Build history of the part. All positions in model axes, mm. A direction names the side the tool comes from. Round coordinates to 2 decimals unless told otherwise and drop trailing zeros. Write each loop counter-clockwise with the first axis right and the second up, starting at its lowest first coordinate (ties: lowest second). Pieces come first, ordered by that corner, then holes. Notation, with made-up numbers: (-7, 85) - (42, 85) arc R8 cw to (42, 93) - close; hole circle Ø3 at (61, 52.25). An arc over 180 degrees is marked (long way). Answer as a JSON object with one key per item and string values. Group by question number.
Item 1: Slice it at A-A, the plane y = 11. List the corners of the cut face in (x, z), then the cut area to 3 significant figures.
Item 2: Flat gauge pins, fed straight in: pin 1 (3.5 mm diameter, centred on x = 11, y = 0, fed in from -Z); pin 2 (8 mm diameter, centred on x = 2, y = -0.5, fed in from +Z); pin 3 (3.5 mm diameter, centred on x = -11, y = 0, fed in from +Z); pin 4 (1.5 mm diameter, centred on x = -5.5, z = 0.5, fed in from +Y). Where does each tip first touch, or does it go through?
Item 3: Probe line 1 (Y direction, x = 0, z = 1.1); line 2 (Y direction, x = -1.5, z = 2.15); line 3 (Y direction, x = -8.75, z = 0.35). List the from-to ranges inside material, lowest first. Write a range as from..to.
Item 4: Two-plate mould, pull along Y, no slides. Class faces 1 (the flat face through (6, 0, 3)), 2 (the cylindrical face through (-14.985, 0.66, 1.479)), 3 (the cylindrical face through (-0.54, 13.44, 1.24)): +Y half, -Y half, draft (parallel to the pull), parting line (faces both ways), or undercut.
Item 5: Which spindle directions (+Z, -Z, +X, -X, +Y, -Y) get a long thin tool onto all of the face, cutting with end or side? Do faces 4 (the cylindrical face through (-1.08, -4.88, 2.25)), 5 (the cylindrical face through (-0.54, -8.56, 1.24)), 6 (the cylindrical face through (-0.54, -2.44, 1.01)). Say none if no direction does.
Item 6: Slice it at C-C, the plane y = 0. Give the number of separate pieces and of enclosed holes in the cut face, then the cut area to 3 significant figures.
from build123d import *

# Parameters (mm, degrees)
SKETCH_R        = 15
SKETCH_R_2      = 1.5
PAD_DEPTH       = 3
SKETCH002_R     = 2.5
POCKET_DEPTH    = 9
SKETCH001_R     = 5
POCKET001_DEPTH = 1
SKETCH003_R     = 2.5
POCKET002_DEPTH = 2
CHAMFER_SIZE    = 0.5
CHAMFER001_SIZE = 0.4


with BuildPart() as part:
    # Sketch → Pad (new body)
    with BuildSketch(Plane.XY):
        Circle(SKETCH_R)
        with Locations((0, 11)):
            Circle(SKETCH_R_2, mode=Mode.SUBTRACT)
        with Locations((-11, 0)):
            Circle(SKETCH_R_2, mode=Mode.SUBTRACT)
        with Locations((0, -11)):
            Circle(SKETCH_R_2, mode=Mode.SUBTRACT)
        with Locations((11, 0)):
            Circle(SKETCH_R_2, mode=Mode.SUBTRACT)
    extrude(amount=PAD_DEPTH)

    # Sketch002 (on Face7 of Pad) → Pocket (cut)
    with BuildSketch(Plane.XY.offset(3)):
        Circle(SKETCH002_R)
    extrude(amount=-POCKET_DEPTH, mode=Mode.SUBTRACT)

    # Sketch001 (on Face7 of Pad) → Pocket001 (cut)
    with BuildSketch(Plane.XY.offset(3)):
        Circle(SKETCH001_R)
    extrude(amount=-POCKET001_DEPTH, mode=Mode.SUBTRACT)

    # Sketch003 (on Face2 of Pocket001) → Pocket002 (cut)
    with BuildSketch(Plane(origin=(0, 0, 0), x_dir=(1, 0, 0), z_dir=(0, 0, -1))):
        with Locations((0, 11)):
            Circle(SKETCH003_R)
        with Locations((11, 0)):
            Circle(SKETCH003_R)
        with Locations((0, -11)):
            Circle(SKETCH003_R)
        with Locations((-11, 0)):
            Circle(SKETCH003_R)
    extrude(amount=-POCKET002_DEPTH, mode=Mode.SUBTRACT)

    # Chamfer
    chamfer_edges = [part.edges().sort_by_distance(p)[0] for p in [
        (-1.5, 11, 3),
        (9.5, 0, 3),
        (-1.5, -11, 3),
        (-12.5, 0, 3),
        (-5, 0, 3),
        (-2.5, 0, 2),
        (-2.5, -11, 0),
        (8.5, 0, 0),
        (-2.5, 11, 0),
        (-13.5, 0, 0),
        (-2.5, 0, 0),
    ]]
    chamfer(chamfer_edges, length=CHAMFER_SIZE)

    # Chamfer001
    chamfer001_edges = [part.edges().sort_by_distance(p)[0] for p in [
        (-1.5, -11, 2),
        (9.5, 0, 2),
        (-1.5, 11, 2),
        (-12.5, 0, 2),
    ]]
    chamfer(chamfer001_edges, length=CHAMFER001_SIZE)


solid = part.part
Geometry says:
{
 "1": {"outline": "(-10.2, 0) - (-3, 0) - (-2.5, 0.5) - (-2.5, 2) - (-1.9, 2) - (-1.5, 2.4) - (-1.5, 2.5) - (-2, 3) - (-10.2, 3) - close; (1.5, 2.4) - (1.9, 2) - (2.5, 2) - (2.5, 0.5) - (3, 0) - (10.2, 0) - (10.2, 3) - (2, 3) - (1.5, 2.5) - close", "area": "47.5 mm^2"},
 "2": {"pin 1": "stops at z = 2.15", "pin 2": "stops at z = 3", "pin 3": "stops at z = 2.75", "pin 4": "stops at y = 14.23"},
 "3": {"line 1": "y = -15..-13.5, -8.5..-2.5, 2.5..8.5, 13.5..15", "line 2": "y = -14.92..-11.9, -10.1..-4.77, 4.77..10.1, 11.9..14.92", "line 3": "y = -12.18..-1.4, 1.4..12.18"},
 "4": {"face 1": "draft", "face 2": "parting line", "face 3": "undercut"},
 "5": {"face 4": "+Z", "face 5": "-Z", "face 6": "+Z, -Z"},
 "6": {"separate pieces": "4", "enclosed holes": "0", "area": "41.9 mm^2"}
}
